Design review of the part built by this model. Coordinates are the model's own, in mm. Give positions to 0.01 mm unless a question says otherwise; leave off trailing zeros. Order: outer loops, then holes, each group sorted by start corner. A loop starts at its lowest first (then second) coordinate and runs counter-clockwise, first axis right, second up. Notation, with made-up numbers: (-25.5, 83) -> (9.5, 83) arc R13 ccw to (9.5, 89) -> close; hole circle Ø7 at (84.25, 69). An arc over 180 degrees is marked (long way). Use a Markdown table: item, result. Add a question column.
Autodesk Inventor part; units mm, degrees
ref_plane "YZ Plane" through (0, 0, 0) normal (1, 0, 0) x (0, 1, 0)
ref_plane "XZ Plane" through (0, 0, 0) normal (0, 1, 0) x (-1, 0, 0)
ref_plane "XY Plane" through (0, 0, 0) normal (0, 0, 1) x (1, 0, 0)
sketch "Sketch1" plane through (0, 0, 0) normal (0, 0, 1) x (1, 0, 0)
  line L0 (-75.565, 0) -> (75.565, 0)
  line L1 (0, -76.9938) -> (0, 84.1375)
  circle A0 centre (0, 0) radius 53.975 construction
  arc A1 (28.575, 46.7235) -> (-28.575, 46.7235) centre (0, 0) ccw
  arc A2 (28.575, 54.0275) -> (-28.575, 54.0275) centre (0, 0) ccw
  line L2 (-28.575, 46.7235) -> (-28.575, 54.0275)
  line L3 (28.575, 46.7235) -> (28.575, 54.0275)
  dimension "d0" = 107.95
  dimension "d1" = 0.7937
  dimension "d2" = 6.35
  dimension "d3" = 57.15
extrude "Extrusion1" add sketch "Sketch1" along normal blind 6.35
sketch "Sketch2" plane through (0, 0, 6.35) normal (0, 0, 1) x (1, 0, 0)
  line L0 (-28.575, 46.7235) -> (-28.575, 54.0275)
  arc A0 (28.575, 46.7235) -> (-28.575, 46.7235) centre (0, 0) ccw
  line L1 (28.575, 54.0275) -> (28.575, 46.7235)
  point P0 (25.4, 51.9032)
  point P1 (-25.4, 51.9032)
  dimension "d6" = 3.175
  dimension "d7" = 3.175
  dimension "d8" = 57.785
hole "Hole1" at (25.4, 51.9032, 6.35) at (-25.4, 51.9032, 6.35) direction (0, 0, -1) diameter 3.175 end through all
properties part number "motor stay top"
1) The part is to be moulded in two halves that separate along Y. For faces 1 (the cylindrical face through (-0.416, 61.117, 3.131)), 2 (the flat face through (0, 56, 0)), 3 (the cylindrical face through (-26.473, 53.073, 3.131)), 4 (the cylindrical face through (25.33, 53.49, 3.13)), say which applies: +Y half, -Y half, draft (parallel to the pull), parting line (faces both ways), or undercut.
2) Add section D-D (x = 12). Give the boundary of the cut face in (y, z), then the cut area to 3 significant figures.
3) Add section A-A (y = 49.5). Give the boundary of the cut face in (x, z) (3 decimals).
4) For L1, parallel to Y at x = -25.4, z = 4.25; L2, parallel to Y at x = -0.5, z = 3.5; L3, parallel to X at y = 50.5, z = 3.5 (3 decimals), list the stretches that pass through material, from the lowest coordinate up. Write a range as [from, to].
5) Insertion check: pin 1 (3 mm diameter, centred on x = -18.5, z = 2.5, fed in from +Y); pin 2 (3 mm diameter, centred on x = -6, z = 5.5, fed in from +Y); pin 3 (1.9 mm diameter, centred on x = 25.4, y = 51.9, fed in from -Z); pin 4 (1 mm diameter, centred on x = 17, z = 3.5, fed in from +Y). Each pin has a flat end and moves straight along its axis. Give the tip position at first contact, or say it passes through.
6) Add section C-C (z = 0.75). Give the boundary of the cut face in (x, y) (1 decimal).
7) Add section B-B (x = -25.4). Give the boundary of the cut face in (y, z), then the cut area to 3 significant figures.
Worked answers:
| question | item | result |
|---|---|---|
| 1 | face 1 | +Y half |
| 1 | face 2 | draft |
| 1 | face 3 | undercut |
| 1 | face 4 | undercut |
| 2 | outline | (53.44, 0) -> (59.93, 0) -> (59.93, 6.35) -> (53.44, 6.35) -> close |
| 2 | area | 41.2 mm^2 |
| 3 | outline | (-28.575, 0) -> (-23.439, 0) -> (-23.439, 6.35) -> (-28.575, 6.35) -> close; (23.439, 0) -> (28.575, 0) -> (28.575, 6.35) -> (23.439, 6.35) -> close |
| 4 | L1 | [48.52, 50.32], [53.49, 55.59] |
| 4 | L2 | [54.77, 61.12] |
| 4 | L3 | [-28.575, -26.142], [-24.658, -21.198], [21.198, 24.658], [26.142, 28.575] |
| 5 | pin 1 | y = 58.71 |
| 5 | pin 2 | y = 60.95 |
| 5 | pin 3 | through |
| 5 | pin 4 | y = 58.85 |
| 6 | outline | (-28.6, 46.7) arc R54.8 cw to (28.6, 46.7) -> (28.6, 54) arc R61.1 ccw to (-28.6, 54) -> close; hole circle Ø3.2 at (-25.4, 51.9); hole circle Ø3.2 at (25.4, 51.9) |
| 7 | outline | (48.52, 0) -> (50.32, 0) -> (50.32, 6.35) -> (48.52, 6.35) -> close; (53.49, 0) -> (55.59, 0) -> (55.59, 6.35) -> (53.49, 6.35) -> close |
| 7 | area | 24.7 mm^2 |
